```python
from build123d import *

# Parameters (mm, degrees)
SKETCH1_R           = 14.1
BOSS_EXTRUDE1_DEPTH = 3
CUT_EXTRUDE1_DEPTH  = 4


with BuildPart() as part:
    # Sketch1 → Boss-Extrude1 (new body)
    with BuildSketch(Plane(origin=(0, 0, 0), x_dir=(1, 0, 0), z_dir=(0, 1, 0))):
        with BuildLine():
            Line((3.491378029, 30.5), (-3.491378029, 30.5))
            ThreePointArc((-3.491378029, 30.5), (-5.40479519, 30.119397663), (-7.026911935, 29.035533906))
            Line((-7.026911935, 29.035533906), (-29.035533906, 7.026911935))
            ThreePointArc((-29.035533906, 7.026911935), (-30.119397663, 5.40479519), (-30.5, 3.491378029))
            Line((-30.5, 3.491378029), (-30.5, -3.491378029))
            ThreePointArc((-30.5, -3.491378029), (-30.119397663, -5.40479519), (-29.035533906, -7.026911935))
            Line((-29.035533906, -7.026911935), (-7.026911935, -29.035533906))
            ThreePointArc((-7.026911935, -29.035533906), (-5.40479519, -30.119397663), (-3.491378029, -30.5))
            Line((-3.491378029, -30.5), (3.491378029, -30.5))
            ThreePointArc((3.491378029, -30.5), (5.40479519, -30.119397663), (7.026911935, -29.035533906))
            Line((7.026911935, -29.035533906), (29.035533906, -7.026911935))
            ThreePointArc((29.035533906, -7.026911935), (30.119397662, -5.404795191), (30.5, -3.491378029))
            Line((30.5, -3.491378029), (30.5, 3.491378029))
            ThreePointArc((30.5, 3.491378029), (30.119397662, 5.40479519), (29.035533906, 7.026911934))
            Line((29.035533906, 7.026911934), (7.026911934, 29.035533906))
            ThreePointArc((7.026911934, 29.035533906), (5.40479519, 30.119397662), (3.491378029, 30.5))
        make_face()
        Circle(SKETCH1_R, mode=Mode.SUBTRACT)
    extrude(amount=BOSS_EXTRUDE1_DEPTH)

    # Sketch2 → Cut-Extrude1 (cut, through all)
    with BuildSketch(Plane(origin=(0, 3, 0), x_dir=(1, 0, 0), z_dir=(0, 1, 0))):
        Polygon((-26.25, 7.929437252), (-26.25, 6.129437252), (-24.9, 6.129437252), (-24.9, 4.779437252), (-23.1, 4.779437252), (-23.1, 6.129437252), (-21.75, 6.129437252), (-21.75, 7.929437252), (-23.1, 7.929437252), (-23.1, 9.279437252), (-24.9, 9.279437252), (-24.9, 7.929437252), align=None)
        Polygon((-23.1, -4.779437252), (-24.9, -4.779437252), (-24.9, -6.129437252), (-26.25, -6.129437252), (-26.25, -7.929437252), (-24.9, -7.929437252), (-24.9, -9.279437252), (-23.1, -9.279437252), (-23.1, -7.929437252), (-21.75, -7.929437252), (-21.75, -6.129437252), (-23.1, -6.129437252), align=None)
        Polygon((7.929437252, 23.1), (9.279437252, 23.1), (9.279437252, 24.9), (7.929437252, 24.9), (7.929437252, 26.25), (6.129437252, 26.25), (6.129437252, 24.9), (4.779437252, 24.9), (4.779437252, 23.1), (6.129437252, 23.1), (6.129437252, 21.75), (7.929437252, 21.75), align=None)
        Polygon((26.25, -7.929437252), (26.25, -6.129437252), (24.9, -6.129437252), (24.9, -4.779437252), (23.1, -4.779437252), (23.1, -6.129437252), (21.75, -6.129437252), (21.75, -7.929437252), (23.1, -7.929437252), (23.1, -9.279437252), (24.9, -9.279437252), (24.9, -7.929437252), align=None)
        Polygon((-4.779437252, 24.9), (-6.129437252, 24.9), (-6.129437252, 26.25), (-7.929437252, 26.25), (-7.929437252, 24.9), (-9.279437252, 24.9), (-9.279437252, 23.1), (-7.929437252, 23.1), (-7.929437252, 21.75), (-6.129437252, 21.75), (-6.129437252, 23.1), (-4.779437252, 23.1), align=None)
        Polygon((26.25, 7.929437252), (24.9, 7.929437252), (24.9, 9.279437252), (23.1, 9.279437252), (23.1, 7.929437252), (21.75, 7.929437252), (21.75, 6.129437252), (23.1, 6.129437252), (23.1, 4.779437252), (24.9, 4.779437252), (24.9, 6.129437252), (26.25, 6.129437252), align=None)
        Polygon((-6.129437252, -26.25), (-6.129437252, -24.9), (-4.779437252, -24.9), (-4.779437252, -23.1), (-6.129437252, -23.1), (-6.129437252, -21.75), (-7.929437252, -21.75), (-7.929437252, -23.1), (-9.279437252, -23.1), (-9.279437252, -24.9), (-7.929437252, -24.9), (-7.929437252, -26.25), align=None)
        Polygon((7.929437252, -26.25), (7.929437252, -24.9), (9.279437252, -24.9), (9.279437252, -23.1), (7.929437252, -23.1), (7.929437252, -21.75), (6.129437252, -21.75), (6.129437252, -23.1), (4.779437252, -23.1), (4.779437252, -24.9), (6.129437252, -24.9), (6.129437252, -26.25), align=None)
    extrude(amount=-CUT_EXTRUDE1_DEPTH, mode=Mode.SUBTRACT)


solid = part.part
```
Input: part model. Units: mm. Frame: model coordinates. A direction names the side the tool comes from. Coordinates: 2 decimals unless noted, no trailing zeros. Write each loop counter-clockwise with the first axis right and the second up, starting at its lowest first coordinate (ties: lowest second). Pieces come first, ordered by that corner, then holes. Notation, with made-up numbers: M 23.5,46.25 L 63.5,46.25 A13 ccw 63.5,65.25 Z; hole C 41,18.5 d6. An arc over 180 degrees is marked long. Use one line per item in the form item = value.
Q1. Section A-A (x = 0). Return loops of the section in (y, z).
Answer below:
outline = M 0,-30.5 L 3,-30.5 L 3,-14.1 L 0,-14.1 Z; M 0,14.1 L 3,14.1 L 3,30.5 L 0,30.5 Z
Q2. Material intervals for probe 1 along Z at (x, y) = (0, 1.4); probe 2 along Z at (x, y) = (23, 2.7), sorted ascending. Write a range as from..to.
Answer below:
probe_1 = -30.5..-14.1, 14.1..30.5
probe_2 = -13.06..-7.93, -6.13..6.13, 7.93..13.06
Q3. Draft query along X for faces 3 (the face through (-30.5, 1, 0)), 4 (the face through (26, 2, -6.129)). Return one class per face: released by +X, released by -X, zero draft, split by the parting line, or undercut.
Answer below:
face_3 = released by -X
face_4 = undercut
Q4. Set-up query: faces 1 (the face through (-17.877, 1.479, -18.185)), 2 (the face through (-24.9, 2, -5)). Return all of +Z, -Z, +X, -X, +Y, -Y with unobstructed straight access to the full face (end or side cutting, diameter ignored); none if empty.
Answer below:
face_1 = -Z, -X, +Y, -Y
face_2 = +Y, -Y
Q5. Section B-B (z = 0). Return loops of the section in (x, y), plus the area to 3 significant figures.
Answer below:
outline = M -30.5,0 L -14.1,0 L -14.1,3 L -30.5,3 Z; M 14.1,0 L 30.5,0 L 30.5,3 L 14.1,3 Z
area = 98.4 mm²
Q6. First-contact query: pin 1 (0.7 mm diameter, centred on y = 2, z = 26, fed in from -X); pin 2 (0.5 mm diameter, centred on y = 1, z = 23.5, fed in from -X); pin 3 (1.5 mm diameter, centred on y = 1, z = 8.5, fed in from +X). Flat tips, straight axial feed; report the tip coordinate or a pass-through.
Answer below:
pin_1 = -10.41
pin_2 = -12.81
pin_3 = 28.31
Q7. Section D-D (x = 19). Return loops of the section in (y, z), plus the area to 3 significant figures.
Answer below:
outline = M 0,-17.06 L 3,-17.06 L 3,17.06 L 0,17.06 Z
area = 102 mm²
Q8. Section C-C (y = 1.3). Count the separate pieces of the cut face and the enclosed holes in it, plus the area to 3 significant figures.
Answer below:
separate_pieces = 1
enclosed_holes = 9
area = 1,740 mm²
